The model under review builds one solid part; all positions refer to its coordinate system, in mm. Coordinates: 2 decimals unless noted, no trailing zeros. Write each loop counter-clockwise with the first axis right and the second up, starting at its lowest first coordinate (ties: lowest second). Pieces come first, ordered by that corner, then holes.
1) Add section A-A, the plane x = 46.5. State the section outline as (y, z) points.
2) Add section C-C, the plane x = -1. State the section outline as (y, z) points.
3) For P1, Ø1.5, axis at y = 102.5, z = 2, coming from the +X side; P2, Ø3, axis at x = 11, z = 1, coming from the +Y side; P3, Ø3, axis at x = 60, y = 0, coming from the +Z side; P4, Ø1.5, axis at y = 49, z = 3.5, coming from the +X side, all flat-tipped, find the tip position at first contact; note any pin that passes through.
4) For line 1 (Y direction, x = 60, z = 1.65); line 2 (Y direction, x = 48, z = 2.3); line 3 (Y direction, x = -1, z = 2.05), list the stretches that pass through material, from the lowest coordinate up.
5) Add section B-B, the plane y = 0. State the section outline as (x, z) points, then the cut area to 3 significant figures.
6) Add section D-D, the plane z = 3.4. Give the number of separate pieces and of enclosed holes in the cut face, then the cut area to 3 significant figures.
from build123d import *

# Parameters (mm, degrees)
BOSS_EXTRU_1_OUTLINE_W   = 5
BOSS_EXTRU_1_OUTLINE_H   = 5
BOSS_EXTRU_1_OUTLINE_R   = 2
BOSS_EXTRU_1_OUTLINE_R_2 = 2.5
BOSS_EXTRU_1_DEPTH       = 5
CONG_1_R                 = 20
CONG_2_R                 = 40


# Read off the part's stored shape, not the designer's step: Boss.-Extru.1
with BuildPart() as part:
    # Boss.-Extru.1 outline → Boss.-Extru.1 (new body)
    with BuildSketch(Plane.XY):
        with BuildLine():
            Line((10, 10), (10, 90))
            Line((10, 90), (60, 90))
            ThreePointArc((60, 90), (70, 100), (60, 110))
            Line((60, 110), (10, 110))
            Line((10, 110), (10, 190))
            Line((10, 190), (60, 190))
            ThreePointArc((60, 190), (70, 200), (60, 210))
            Line((60, 210), (-20, 210))
            Line((-20, 210), (-20, -10))
            Line((-20, -10), (60, -10))
            ThreePointArc((60, -10), (70, 0), (60, 10))
            Line((60, 10), (10, 10))
        make_face()
        with Locations((-8.5, 77.5)):
            Rectangle(BOSS_EXTRU_1_OUTLINE_W, BOSS_EXTRU_1_OUTLINE_H, mode=Mode.SUBTRACT)
        with Locations((-1, 77.5)):
            Circle(BOSS_EXTRU_1_OUTLINE_R, mode=Mode.SUBTRACT)
        with Locations((-1, 90)):
            Circle(BOSS_EXTRU_1_OUTLINE_R_2, mode=Mode.SUBTRACT)
        with Locations((6.5, 77.5)):
            Rectangle(BOSS_EXTRU_1_OUTLINE_W, BOSS_EXTRU_1_OUTLINE_H, mode=Mode.SUBTRACT)
        with Locations((60, 0)):
            Circle(BOSS_EXTRU_1_OUTLINE_R_2, mode=Mode.SUBTRACT)
        with Locations((-8.5, 102.5)):
            Rectangle(BOSS_EXTRU_1_OUTLINE_W, BOSS_EXTRU_1_OUTLINE_H, mode=Mode.SUBTRACT)
        with Locations((-1, 102.5)):
            Circle(BOSS_EXTRU_1_OUTLINE_R, mode=Mode.SUBTRACT)
        with Locations((6.5, 102.5)):
            Rectangle(BOSS_EXTRU_1_OUTLINE_W, BOSS_EXTRU_1_OUTLINE_H, mode=Mode.SUBTRACT)
        with Locations((60, 100)):
            Circle(BOSS_EXTRU_1_OUTLINE_R_2, mode=Mode.SUBTRACT)
        with Locations((60, 200)):
            Circle(BOSS_EXTRU_1_OUTLINE_R_2, mode=Mode.SUBTRACT)
    extrude(amount=BOSS_EXTRU_1_DEPTH)

    # Congé1
    cong_1_edges = [part.edges().sort_by_distance(p)[0] for p in [
        (10, 10, 2.5),
        (10, 190, 2.5),
        (10, 110, 2.5),
        (10, 90, 2.5),
    ]]
    fillet(cong_1_edges, radius=CONG_1_R)

    # Congé2
    cong_2_edges = [part.edges().sort_by_distance(p)[0] for p in [
        (-20, -10, 2.5),
        (-20, 210, 2.5),
    ]]
    fillet(cong_2_edges, radius=CONG_2_R)


solid = part.part
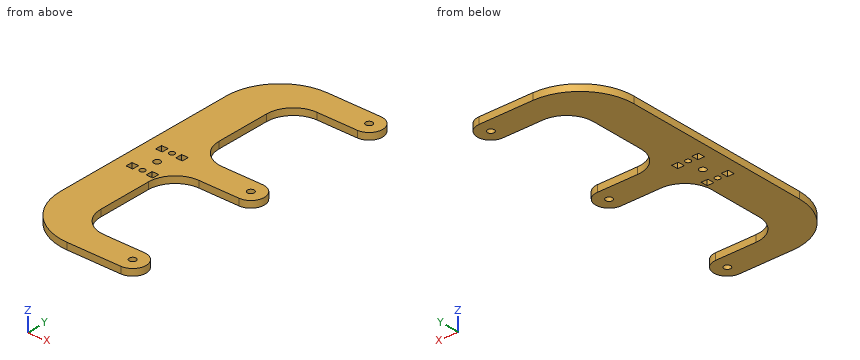
Geometry results:
1. outline: (-10, 0) - (10, 0) - (10, 5) - (-10, 5) - close; (90, 0) - (110, 0) - (110, 5) - (90, 5) - close; (190, 0) - (210, 0) - (210, 5) - (190, 5) - close
2. outline: (-4.04, 0) - (75.5, 0) - (75.5, 5) - (-4.04, 5) - close; (79.5, 0) - (87.5, 0) - (87.5, 5) - (79.5, 5) - close; (92.5, 0) - (100.5, 0) - (100.5, 5) - (92.5, 5) - close; (104.5, 0) - (204.04, 0) - (204.04, 5) - (104.5, 5) - close
3. P1: stops at x = 69.85
3. P2: stops at y = 209.29
3. P3: passes through
3. P4: stops at x = 10
4. line 1: y = -10 to -2.5, 2.5 to 10, 90 to 97.5, 102.5 to 110, 190 to 197.5, 202.5 to 210
4. line 2: y = -10 to 10, 90 to 110, 190 to 210
4. line 3: y = -4.04 to 75.5, 79.5 to 87.5, 92.5 to 100.5, 104.5 to 204.04
5. outline: (-6.46, 0) - (57.5, 0) - (57.5, 5) - (-6.46, 5) - close; (62.5, 0) - (70, 0) - (70, 5) - (62.5, 5) - close
5. area: 357 mm2
6. separate pieces: 1
6. enclosed holes: 10
6. area: 9,520 mm2
